from build123d import *

# Parameters (mm, degrees)
SKETCH1_R           = 3.429
SKETCH1_R_2         = 2.54
BOSS_EXTRUDE1_DEPTH = 3.2004
SKETCH2_R           = 2.413
CUT_EXTRUDE1_DEPTH  = 3.2004
SKETCH5_R           = 1.7272
SKETCH5_W           = 40.894
SKETCH5_H           = 20.32
CUT_EXTRUDE3_DEPTH  = 4.2004
CUT_EXTRUDE5_DEPTH  = 3.2004
SKETCH6_R           = 2.54
CUT_EXTRUDE4_DEPTH  = 4.2004
SKETCH9_R           = 2.159
CUT_EXTRUDE6_DEPTH  = 3.2004
SKETCH10_W          = 107.95
SKETCH10_H          = 3.2512
CUT_EXTRUDE7_DEPTH  = 3.2004
SKETCH11_R          = 3.429
SKETCH11_R_2        = 2.54
CUT_EXTRUDE8_DEPTH  = 3.2004
CUT_EXTRUDE9_DEPTH  = 3.2004
SKETCH15_R          = 2.159
CUT_EXTRUDE10_DEPTH = 3.2004
BOSS_EXTRUDE2_DEPTH = 3.2004
FILLET1_R           = 5.08
CUT_EXTRUDE11_DEPTH = 3.2004
CUT_EXTRUDE12_DEPTH = 3.2004
FILLET2_R           = 12.7


with BuildPart() as part:
    # Sketch1 → Boss-Extrude1 (new body)
    with BuildSketch(Plane.XY):
        with BuildLine():
            Line((0, 0), (120.015, 0))
            ThreePointArc((120.015, 0), (130.351788396, 3.075697789), (137.325636158, 11.302152592))
            Line((137.325636158, 11.302152592), (155.2575, 52.11572))
            ThreePointArc((155.2575, 52.11572), (157.54731739, 67.602183396), (151.630955452, 82.09599151))
            ThreePointArc((151.630955452, 82.09599151), (60.0075, 127.266502568), (-31.615955452, 82.09599151))
            ThreePointArc((-31.615955452, 82.09599151), (-37.53231739, 67.602183396), (-35.2425, 52.11572))
            Line((-35.2425, 52.11572), (-17.310636158, 11.302152592))
            ThreePointArc((-17.310636158, 11.302152592), (-10.336788396, 3.075697789), (0, 0))
        make_face()
        with Locations((120.015, 18.90776)):
            Circle(SKETCH1_R, mode=Mode.SUBTRACT)
        with Locations((0, 18.90776)):
            Circle(SKETCH1_R_2, mode=Mode.SUBTRACT)
        with Locations((19.734727626, 25.566426992)):
            Circle(SKETCH1_R_2, mode=Mode.SUBTRACT)
    extrude(amount=BOSS_EXTRUDE1_DEPTH)

    # Sketch2 → Cut-Extrude1 (cut)
    with BuildSketch(Plane(origin=(0, 0, 0), x_dir=(-1, 0, 0), z_dir=(0, 0, -1))):
        with Locations((-92.0115, 52.11572)):
            Circle(SKETCH2_R)
        with Locations((-76.0095, 52.11572)):
            Circle(SKETCH2_R)
        with Locations((-44.0055, 52.11572)):
            Circle(SKETCH2_R)
        with Locations((-28.0035, 52.11572)):
            Circle(SKETCH2_R)
    extrude(amount=-CUT_EXTRUDE1_DEPTH, mode=Mode.SUBTRACT)

    # Sketch5 → Cut-Extrude3 (cut, through all)
    with BuildSketch(Plane(origin=(0, 0, 0), x_dir=(-1, 0, 0), z_dir=(0, 0, -1))):
        with Locations((-98.932021353, 23.907759967)):
            Circle(SKETCH5_R)
        with Locations((-48.432021353, 13.907760033)):
            Circle(SKETCH5_R)
        with Locations((-48.432021353, 23.907759967)):
            Circle(SKETCH5_R)
        with Locations((-98.932021353, 13.907760033)):
            Circle(SKETCH5_R)
        with Locations((-73.682021353, 18.90776)):
            Rectangle(SKETCH5_W, SKETCH5_H)
    extrude(amount=-CUT_EXTRUDE3_DEPTH, mode=Mode.SUBTRACT)

    # Sketch7 → Cut-Extrude5 (cut)
    with BuildSketch(Plane(origin=(0, 0, 0), x_dir=(-1, 0, 0), z_dir=(0, 0, -1))):
        with BuildLine():
            Line((-98.193021353, 19.92376), (-94.129021353, 19.92376))
            Line((-94.129021353, 19.92376), (-94.129021353, 17.89176))
            Line((-94.129021353, 17.89176), (-98.193021353, 17.89176))
            ThreePointArc((-98.193021353, 17.89176), (-99.209021353, 18.90776), (-98.193021353, 19.92376))
        make_face()
        with BuildLine():
            Line((-53.235021353, 19.92376), (-49.171021353, 19.92376))
            ThreePointArc((-49.171021353, 19.92376), (-48.155021353, 18.90776), (-49.171021353, 17.89176))
            Line((-49.171021353, 17.89176), (-53.235021353, 17.89176))
            Line((-53.235021353, 17.89176), (-53.235021353, 19.92376))
        make_face()
    extrude(amount=-CUT_EXTRUDE5_DEPTH, mode=Mode.SUBTRACT)

    # Sketch6 → Cut-Extrude4 (cut, through all)
    with BuildSketch(Plane(origin=(0, 0, 0), x_dir=(-1, 0, 0), z_dir=(0, 0, -1))):
        with Locations((-99.400822485, 30.809360937)):
            Circle(SKETCH6_R)
    extrude(amount=-CUT_EXTRUDE4_DEPTH, mode=Mode.SUBTRACT)

    # Sketch9 → Cut-Extrude6 (cut)
    with BuildSketch(Plane.XY.offset(3.2004)):
        with Locations((21.9075, 3.81)):
            Circle(SKETCH9_R)
        with Locations((60.0075, 3.81)):
            Circle(SKETCH9_R)
        with Locations((98.1075, 3.81)):
            Circle(SKETCH9_R)
    extrude(amount=-CUT_EXTRUDE6_DEPTH, mode=Mode.SUBTRACT)

    # Sketch10 → Cut-Extrude7 (cut)
    with BuildSketch(Plane.XY.offset(3.2004)):
        with Locations((60.0075, 46.68012)):
            Rectangle(SKETCH10_W, SKETCH10_H)
    extrude(amount=-CUT_EXTRUDE7_DEPTH, mode=Mode.SUBTRACT)

    # Sketch11 → Cut-Extrude8 (cut)
    with BuildSketch(Plane.XY.offset(3.2004)):
        with Locations((126.474462556, 80.535782848)):
            Circle(SKETCH11_R)
        with Locations((105.860285087, 92.437383759)):
            Circle(SKETCH11_R_2)
    extrude(amount=-CUT_EXTRUDE8_DEPTH, mode=Mode.SUBTRACT)

    # Sketch14 → Cut-Extrude9 (cut)
    with BuildSketch(Plane(origin=(0, 0, 0), x_dir=(-1, 0, 0), z_dir=(0, 0, -1))):
        with BuildLine():
            Line((-44.300963253, 126.193661773), (-33.301235987, 102.993397816))
            Line((-33.301235987, 102.993397816), (25.933073592, 73.679154431))
            Line((25.933073592, 73.679154431), (30.688377769, 83.288038279))
            ThreePointArc((30.688377769, 83.288038279), (-2.643821722, 112.015909409), (-44.300963253, 126.193661773))
        make_face()
    extrude(amount=-CUT_EXTRUDE9_DEPTH, mode=Mode.SUBTRACT)

    # Sketch15 → Cut-Extrude10 (cut)
    with BuildSketch(Plane.XY.offset(3.2004)):
        with Locations((8.255, 18.90776)):
            Circle(SKETCH15_R)
        with Locations((109.47654, 18.90776)):
            Circle(SKETCH15_R)
    extrude(amount=-CUT_EXTRUDE10_DEPTH, mode=Mode.SUBTRACT)

    # Sketch16 → Boss-Extrude2 (add)
    with BuildSketch(Plane.XY.offset(3.2004)):
        with BuildLine():
            Line((-45.041102147, 54.757414103), (-19.827237301, 11.4051976))
            ThreePointArc((-19.827237301, 11.4051976), (-11.436759498, 3.05471175), (0, 0))
            ThreePointArc((0, 0), (-15.87467945, 35.815989499), (-25.933073592, 73.679154431))
            Line((-25.933073592, 73.679154431), (-33.949803194, 89.878291377))
            ThreePointArc((-33.949803194, 89.878291377), (-38.093703484, 85.921735268), (-42.068546328, 81.795372437))
            ThreePointArc((-42.068546328, 81.795372437), (-48.007013112, 68.765867356), (-45.041102147, 54.757414103))
        make_face()
    extrude(amount=-BOSS_EXTRUDE2_DEPTH)

    # Fillet1
    fillet1_edges = [part.edges().sort_by_distance(p)[0] for p in [
        (44.300963253, 126.193661773, 1.6002),
        (-33.949803194, 89.878291377, 1.6002),
    ]]
    fillet(fillet1_edges, radius=FILLET1_R)

    # Sketch17 → Cut-Extrude11 (cut)
    with BuildSketch(Plane(origin=(0, 0, 0), x_dir=(-1, 0, 0), z_dir=(0, 0, -1))):
        with BuildLine():
            Line((-34.3535, 67.35572), (-21.6535, 67.35572))
            ThreePointArc((-21.6535, 67.35572), (-18.4785, 64.18072), (-21.6535, 61.00572))
            Line((-21.6535, 61.00572), (-34.3535, 61.00572))
            ThreePointArc((-34.3535, 61.00572), (-37.5285, 64.18072), (-34.3535, 67.35572))
        make_face()
    extrude(amount=-CUT_EXTRUDE11_DEPTH, mode=Mode.SUBTRACT)

    # Sketch18 → Cut-Extrude12 (cut)
    with BuildSketch(Plane(origin=(0, 0, 0), x_dir=(-1, 0, 0), z_dir=(0, 0, -1))):
        Polygon((25.933073592, 73.679154431), (45.392963589, 113.00110224), (91.414081971, 83.705991697), (68.906880725, 52.412009588), align=None)
    extrude(amount=-CUT_EXTRUDE12_DEPTH, mode=Mode.SUBTRACT)

    # Fillet2
    fillet2_edges = [part.edges().sort_by_distance(p)[0] for p in [
        (-47.882876097, 62.816499705, 1.6002),
    ]]
    fillet(fillet2_edges, radius=FILLET2_R)


solid = part.part
The listing builds one solid part. Answer for the finished solid, in the listing's coordinates (mm). Round coordinates to 2 decimals unless told otherwise and drop trailing zeros. Write each loop counter-clockwise with the first axis right and the second up, starting at its lowest first coordinate (ties: lowest second). Pieces come first, ordered by that corner, then holes. Notation, with made-up numbers: (-21.5, 41.25) - (-7.5, 41.25) arc R9 cw to (-7.5, 58.25) - close; hole circle Ø5 at (-11.5, -33). An arc over 180 degrees is marked (long way). Use a Markdown table: item, result. Add a question column.
1. Consider line 1 (X direction, y = 18, z = 0.85); line 2 (Y direction, x = 64.5, z = 2.25); line 3 (Y direction, x = 90.5, z = 2.9). Determine where each line is inside the solid, lowest interval first.
2. The part is cut by section B-B (z = 1.15). Give the number of separate pieces and of enclosed holes in the cut face, and give its area (3 significant figures).
3. The part is cut by section A-A (y = 3.81). Write down the section's boundary in (x, z).
4. Flat-ended cylindrical pins translate along their axes: P1, Ø1.6, axis at y = 11.5, z = 2, coming from the +X side; P2, Ø1.5, axis at y = 44, z = 0.5, coming from the -X side; P3, Ø4.5, axis at x = 0, y = 18.91, coming from the +Z side; P4, Ø1.6, axis at x = 96, z = 2, coming from the +Y side. Find the tip coordinate at first contact, or state that the pin passes through.
5. For a pull along X with two mould halves and no side action, classify faces 1 (the face through (98.035, 32.951, 1.578)), 2 (the face through (-31.315, 31.158, 1.623)), 3 (the face through (130.22, 2.99, 1.58)) as +X half, -X half, draft (parallel to the pull), parting line (faces both ways), or undercut.
6. The part is cut by section C-C (x = -16). Write down the section's boundary in (y, z).
Reported:
| question | item | result |
|---|---|---|
| 1 | line 1 | -23.66 to -2.37, 2.37 to 6.3, 10.21 to 48.71, 98.65 to 107.52, 111.44 to 116.71, 123.32 to 140.27 |
| 1 | line 2 | 0 to 8.75, 29.07 to 45.05, 48.31 to 127.18 |
| 1 | line 3 | 0 to 8.75, 29.07 to 45.05, 48.31 to 50.23, 54 to 123.17 |
| 2 | separate pieces | 1 |
| 2 | enclosed holes | 22 |
| 2 | area | 17,300 mm^2 |
| 3 | outline | (-12.66, 0) - (19.75, 0) - (19.75, 3.2) - (-12.66, 3.2) - close; (24.07, 0) - (57.85, 0) - (57.85, 3.2) - (24.07, 3.2) - close; (62.17, 0) - (95.95, 0) - (95.95, 3.2) - (62.17, 3.2) - close; (100.27, 0) - (131.4, 0) - (131.4, 3.2) - (100.27, 3.2) - close |
| 4 | P1 | x = 137.76 |
| 4 | P2 | x = -39.22 |
| 4 | P3 | through |
| 4 | P4 | y = 121.77 |
| 5 | face 1 | undercut |
| 5 | face 2 | -X half |
| 5 | face 3 | +X half |
| 6 | outline | (6.5, 0) - (78.59, 0) - (78.59, 3.2) - (6.5, 3.2) - close |
